For this review, take the finished solid that the model builds, in its own axes (mm). A direction names the side the tool comes from. Give positions to 0.01 mm unless a question says otherwise; leave off trailing zeros. Write each loop counter-clockwise with the first axis right and the second up, starting at its lowest first coordinate (ties: lowest second). Pieces come first, ordered by that corner, then holes. Notation, with made-up numbers: M 49,16 L 57,16 A37 cw 57,52 Z; hole C 43.25,10.25 d10. An arc over 180 degrees is marked long. Write item = value, one per line.
```python
from build123d import *

# Parameters (mm, degrees)
SKETCH1_W           = 74
SKETCH1_H           = 30
BOSS_EXTRUDE1_DEPTH = 5.75
SKETCH2_W           = 9.25
SKETCH2_H           = 30
BOSS_EXTRUDE2_DEPTH = 2.25
SKETCH3_R           = 2
CUT_EXTRUDE1_DEPTH  = 9


with BuildPart() as part:
    # Sketch1 → Boss-Extrude1 (new body)
    with BuildSketch(Plane(origin=(0, 0, 0), x_dir=(1, 0, 0), z_dir=(0, 1, 0))):
        with Locations((37, 15)):
            Rectangle(SKETCH1_W, SKETCH1_H)
    extrude(amount=BOSS_EXTRUDE1_DEPTH)

    # Sketch2 → Boss-Extrude2 (add)
    with BuildSketch(Plane(origin=(0, 5.75, 0), x_dir=(1, 0, 0), z_dir=(0, 1, 0))):
        with Locations((4.625, 15)):
            Rectangle(SKETCH2_W, SKETCH2_H)
        with Locations((69.375, 15)):
            Rectangle(SKETCH2_W, SKETCH2_H)
    extrude(amount=BOSS_EXTRUDE2_DEPTH)

    # Sketch3 → Cut-Extrude1 (cut, through all)
    with BuildSketch(Plane(origin=(0, 0, 0), x_dir=(-1, 0, 0), z_dir=(0, -1, 0))):
        with Locations((-68, 10)):
            Circle(SKETCH3_R)
        with Locations((-6, 10)):
            Circle(SKETCH3_R)
    extrude(amount=-CUT_EXTRUDE1_DEPTH, mode=Mode.SUBTRACT)


solid = part.part
```
1. The part is to be moulded in two halves that separate along Z. For faces 3 (the face through (6, 4, -12)), 4 (the face through (0, 4, -15)), 5 (the face through (36, 3, 0)), say which applies: +Z half, -Z half, draft (parallel to the pull), parting line (faces both ways), or undercut.
Responses:
face_3 = undercut
face_4 = draft
face_5 = +Z half
2. We need section D-D, the plane x = 53. Write out the cut boundary in (y, z).
Responses:
outline = M 0,-30 L 5.75,-30 L 5.75,0 L 0,0 Z
3. We need section B-B, the plane z = -10. Write out the cut boundary in (x, y).
Responses:
outline = M 0,0 L 4,0 L 4,8 L 0,8 Z; M 8,0 L 66,0 L 66,8 L 64.75,8 L 64.75,5.75 L 9.25,5.75 L 9.25,8 L 8,8 Z; M 70,0 L 74,0 L 74,8 L 70,8 Z
4. We need section C-C, the plane z = -18.5. Write out the cut boundary in (x, y).
Responses:
outline = M 0,0 L 74,0 L 74,8 L 64.75,8 L 64.75,5.75 L 9.25,5.75 L 9.25,8 L 0,8 Z
5. We need section A-A, the plane x = 6. Write out the cut boundary in (y, z), then the cut area to 3 significant figures.
Responses:
outline = M 0,-30 L 8,-30 L 8,-12 L 0,-12 Z; M 0,-8 L 8,-8 L 8,0 L 0,0 Z
area = 208 mm2
6. Insertion check: P1, Ø15, axis at x = 45, z = -17, coming from the +Y side; P2, Ø2.5, axis at x = 6, z = -10, coming from the -Y side. Each pin has a flat end and moves straight along its axis. Give the tip position at first contact, or say it passes through.
Responses:
P1 = 5.75
P2 = through
7. Machinability: for faces 1 (the face through (66.092, 3.944, -10.601)), 2 (the face through (37, 5.75, -15)), which of the approach directions +Z, -Z, +X, -X, +Y, -Y give a long, thin tool a straight path to every point of the face, cutting with its end or side? Answer none if there is none.
Responses:
face_1 = +Y, -Y
face_2 = +Z, -Z, +Y
8. For line 1 along X through (y, z) = (5, -10); line 2 along Z through (x, y) = (68, 6.75); line 3 along X through (y, z) = (2.75, -11.5), list the stretches that pass through material, from the lowest coordinate up. Write a range as from..to.
Responses:
line_1 = 0..4, 8..66, 70..74
line_2 = -30..-12, -8..0
line_3 = 0..4.68, 7.32..66.68, 69.32..74
